from build123d import *

# Parameters (mm, degrees)
SKETCH_D_W               = 44.2
SKETCH_D_H               = 120
BOSS_EXTRUDE1_DEPTH      = 3
M3_CLEARANCE_HOLE1_D     = 3.4
M3_CLEARANCE_HOLE1_DEPTH = 15
M3_CLEARANCE_HOLE1_TIP   = 1.021463052
SKETCH6_W                = 8
SKETCH6_H                = 35
CUT_EXTRUDE1_DEPTH       = 75.008813719
FILLET1_R                = 3.5


with BuildPart() as part:
    # Sketch d → Boss-Extrude1 (new body)
    with BuildSketch(Plane.XY):
        with Locations((0.312368929, 10.469782369)):
            Rectangle(SKETCH_D_W, SKETCH_D_H)
    extrude(amount=BOSS_EXTRUDE1_DEPTH)

    # M3 Clearance Hole1
    with Locations(Plane.XY.offset(3)):
        with Locations((-18.787631071, 53.469782369), (-18.787631071, 38.469782369), (-18.787631071, -19.530217631), (-18.787631071, -34.530217631), (19.412368929, -34.530217631), (19.412368929, -19.530217631), (19.412368929, 38.469782369), (19.412368929, 53.469782369)):
            Hole(M3_CLEARANCE_HOLE1_D / 2, depth=M3_CLEARANCE_HOLE1_DEPTH)
            with Locations((0, 0, -(M3_CLEARANCE_HOLE1_DEPTH + M3_CLEARANCE_HOLE1_TIP / 2))):  # 118° drill point
                Cone(0, M3_CLEARANCE_HOLE1_D / 2, M3_CLEARANCE_HOLE1_TIP, mode=Mode.SUBTRACT)

    # Sketch6 → Cut-Extrude1 (cut, through all)
    with BuildSketch(Plane.XY.offset(3)):
        with Locations((-17.787631071, 9.469782369)):
            Rectangle(SKETCH6_W, SKETCH6_H)
    extrude(amount=-CUT_EXTRUDE1_DEPTH, mode=Mode.SUBTRACT)

    # Fillet1
    fillet1_edges = [part.edges().sort_by_distance(p)[0] for p in [
        (-21.787631071, -8.030217631, 1.5),
        (-21.787631071, 26.969782369, 1.5),
        (-13.787631071, 26.969782369, 1.5),
        (-13.787631071, -8.030217631, 1.5),
    ]]
    fillet(fillet1_edges, radius=FILLET1_R)


solid = part.part
Work out the finished part from the listing and answer in its coordinate system (mm). A direction names the side the tool comes from. Coordinates: 2 decimals unless noted, no trailing zeros. Write each loop counter-clockwise with the first axis right and the second up, starting at its lowest first coordinate (ties: lowest second). Pieces come first, ordered by that corner, then holes. Notation, with made-up numbers: M 30.25,-26 L 79.25,-26 A18 ccw 79.25,3 Z; hole C -17.5,34 d4. An arc over 180 degrees is marked long. Use one line per item in the form item = value. Start each with the question number.
1. The mould has two halves that part along Y. Classify faces 3 (the face through (0, 11, 0)), 4 (the face through (-13.788, 9, 2)), 5 (the face through (-14.79, 25.92, 1.48)), 6 (the face through (0, 70.47, 1)): released by +Y, released by -Y, zero draft, split by the parting line, or undercut.
2. This flat-tipped pin is pushed along its axis until it touches: P1, Ø3, axis at x = -17, y = 10, coming from the +Z side. Where does it stop, or does it pass through?
3. Straight lines are drawn through the part: probe 1 along X at (y, z) = (-33, 2.7); probe 2 along Y at (x, z) = (18, 2.8); probe 3 along X at (y, z) = (3, 1). For each, find the intervals that lie inside material, in ascending order. Write a range as from..to.
4. A tool of negligible diameter and unlimited length cuts with its end or side. For faces 1 (the face through (-20.36, 37.82, 1.48)), 2 (the face through (-20.79, -9.083, 1.479)), from which of +Z, -Z, +X, -X, +Y, -Y can it reach the whole face along a straight path? Write none if from no direction.
5. The part is cut by section B-B (z = 1.95). Give the number of separate pieces and of enclosed holes in the cut face, plus the area to 3 significant figures.
6. The part is cut by section A-A (y = 20). Give the vertices of the cut face in (x, z).
Evaluation:
q1.face_3 = zero draft
q1.face_4 = undercut
q1.face_5 = undercut
q1.face_6 = released by +Y
q2.P1 = through
q3.probe_1 = -21.79..-19.53, -18.05..18.67, 20.15..22.41
q3.probe_2 = -49.53..-35.48, -33.58..-20.48, -18.58..37.52, 39.42..52.52, 54.42..70.47
q3.probe_3 = -13.79..22.41
q4.face_1 = +Z, -Z
q4.face_2 = +Z, -Z, -X
q5.separate_pieces = 1
q5.enclosed_holes = 8
q5.area = 4,950 mm^2
q6.outline = M -13.79,0 L 22.41,0 L 22.41,3 L -13.79,3 Z
